Answer from the drawing. Dimensions are ordinates in mm from the lowest x, y and z of the part. A direction names the side the tool comes from. Give positions to 0.01 mm unless a question says otherwise; leave off trailing zeros. Write each loop counter-clockwise with the first axis right and the second up, starting at its lowest first coordinate (ties: lowest second). Pieces come first, ordered by that corner, then holes.
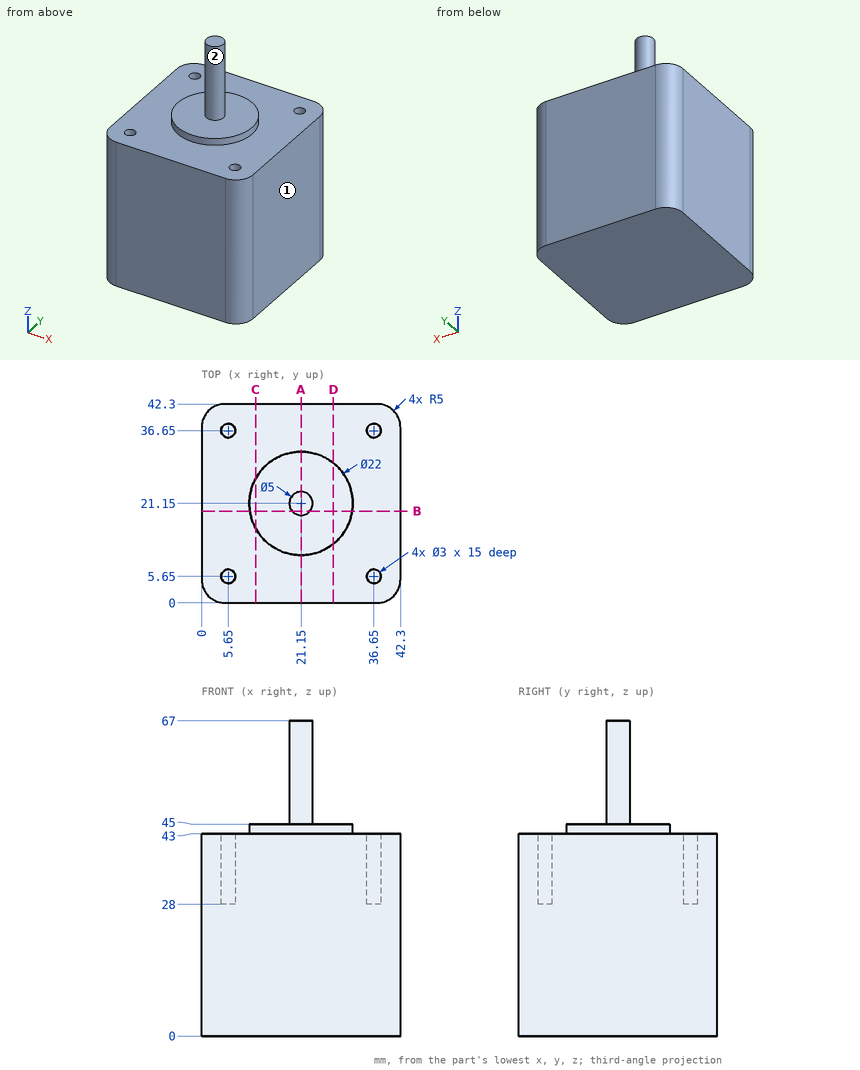
Item 1: Each of these flat-tipped pins is pushed along its axis until it touches: pin 1 Ø2.5 at (x, y) = (6, 36) entering from +Z; pin 2 Ø1.8 at (x, y) = (36.65, 5.65) entering from +Z. Where does it stop, or does it pass through?
Result set:
pin 1: stops at z = 43
pin 2: stops at z = 28
Item 2: Section A-A (x = 21.15) is taken. Write down the section's boundary in (y, z).
Result set:
outline: (0, 0) - (42.3, 0) - (42.3, 43) - (32.15, 43) - (32.15, 45) - (23.65, 45) - (23.65, 67) - (18.65, 67) - (18.65, 45) - (10.15, 45) - (10.15, 43) - (0, 43) - close
Item 3: Find the intervals of material crossed by line 1 along X through (y, z) = (5.65, 37.75); line 2 along Y through (x, z) = (36, 35), in increasing order.
Result set:
line 1: x = 0 to 4.15, 7.15 to 35.15, 38.15 to 42.3
line 2: y = 0 to 4.3, 7 to 35.3, 38 to 42.3
Item 4: Section D-D (x = 28) is taken. Write down the section's boundary in (y, z).
Result set:
outline: (0, 0) - (42.3, 0) - (42.3, 43) - (29.76, 43) - (29.76, 45) - (12.54, 45) - (12.54, 43) - (0, 43) - close
Item 5: Section C-C (x = 11.5) is taken. Write down the section's boundary in (y, z), and give its area (3 significant figures).
Result set:
outline: (0, 0) - (42.3, 0) - (42.3, 43) - (26.43, 43) - (26.43, 45) - (15.87, 45) - (15.87, 43) - (0, 43) - close
area: 1,840 mm2
Item 6: Which of the six approach directions +Z, -Z, +X, -X, +Y, -Y give full straight-line access (tool end or side, diameter ignored) to the marked faces 1 and 2?
Result set:
face 1: +Z, -Z, +X, +Y, -Y
face 2: +Z
Item 7: Section B-B (y = 19.5) is taken. Write down the section's boundary in (x, z).
Result set:
outline: (0, 0) - (42.3, 0) - (42.3, 43) - (32.03, 43) - (32.03, 45) - (23.03, 45) - (23.03, 67) - (19.27, 67) - (19.27, 45) - (10.27, 45) - (10.27, 43) - (0, 43) - close
